```python
from build123d import *

# Parameters (mm, degrees)
SKETCH_R   = 25.426446
SKETCH_R_2 = 1.991345
PAD_DEPTH  = 5


with BuildPart() as part:
    # Sketch → Pad (new body)
    with BuildSketch(Plane.XY):
        Circle(SKETCH_R)
        Circle(SKETCH_R_2, mode=Mode.SUBTRACT)
        with BuildLine():
            Line((-22.250395, 0), (-20.250395, 0))
            ThreePointArc((20.250395, 0), (0, 20.250395), (-20.250395, 0))
            Line((20.250395, 0), (22.250395, 0))
            ThreePointArc((22.250395, 0), (0, 22.250395), (-22.250395, 0))
        make_face(mode=Mode.SUBTRACT)
        with BuildLine():
            ThreePointArc((12.197871, 12.197871), (0, 17.250395), (-12.197871, 12.197871))
            Line((-12.197871, 12.197871), (-10.783657, 10.783657))
            ThreePointArc((10.783657, 10.783657), (0, 15.250395), (-10.783657, 10.783657))
            Line((10.783657, 10.783657), (12.197871, 12.197871))
        make_face(mode=Mode.SUBTRACT)
        with BuildLine():
            Line((10.783657, -10.783657), (12.197871, -12.197871))
            ThreePointArc((-12.197871, -12.197871), (0, -17.250395), (12.197871, -12.197871))
            Line((-12.197871, -12.197871), (-10.783657, -10.783657))
            ThreePointArc((-10.783657, -10.783657), (0, -15.250395), (10.783657, -10.783657))
        make_face(mode=Mode.SUBTRACT)
        with BuildLine():
            ThreePointArc((-4.688023, 11.317889), (-8.662337, 8.662337), (-11.317889, 4.688023))
            Line((-11.317889, 4.688023), (-9.47013, 3.922656))
            ThreePointArc((-3.922656, 9.47013), (-7.248124, 7.248124), (-9.47013, 3.922656))
            Line((-4.688023, 11.317889), (-3.922656, 9.47013))
        make_face(mode=Mode.SUBTRACT)
        with BuildLine():
            ThreePointArc((11.317889, 4.688023), (8.662337, 8.662337), (4.688023, 11.317889))
            Line((4.688023, 11.317889), (3.922656, 9.47013))
            ThreePointArc((9.47013, 3.922656), (7.248124, 7.248124), (3.922656, 9.47013))
            Line((11.317889, 4.688023), (9.47013, 3.922656))
        make_face(mode=Mode.SUBTRACT)
        with BuildLine():
            ThreePointArc((-11.317889, -4.688023), (-8.662337, -8.662337), (-4.688023, -11.317889))
            Line((-4.688023, -11.317889), (-3.922656, -9.47013))
            ThreePointArc((-9.47013, -3.922656), (-7.248124, -7.248124), (-3.922656, -9.47013))
            Line((-11.317889, -4.688023), (-9.47013, -3.922656))
        make_face(mode=Mode.SUBTRACT)
        with BuildLine():
            ThreePointArc((3.922656, -9.47013), (7.248124, -7.248124), (9.47013, -3.922656))
            Line((11.317889, -4.688023), (9.47013, -3.922656))
            ThreePointArc((4.688023, -11.317889), (8.662337, -8.662337), (11.317889, -4.688023))
            Line((4.688023, -11.317889), (3.922656, -9.47013))
        make_face(mode=Mode.SUBTRACT)
        with BuildLine():
            ThreePointArc((0, 7.250395), (-7.250395, 0), (0, -7.250395))
            Line((0, -5.250395), (0, -7.250395))
            ThreePointArc((0, 5.250395), (-5.250395, 0), (0, -5.250395))
            Line((0, 7.250395), (0, 5.250395))
        make_face(mode=Mode.SUBTRACT)
    extrude(amount=PAD_DEPTH)


solid = part.part
```
Model file for the job. Use its own axes, mm. Give positions to 0.01 mm unless a question says otherwise; leave off trailing zeros. Order: outer loops, then holes, each group sorted by start corner. A loop starts at its lowest first (then second) coordinate and runs counter-clockwise, first axis right, second up.
1) Pin check, flat tips, straight feed: pin 1 (3 mm diameter, centred on x = -1, z = 3.5, fed in from +Y); pin 2 (1.6 mm diameter, centred on y = 6.5, z = 3.5, fed in from -X); pin 3 (1 mm diameter, centred on x = -21.5, z = 3, fed in from +Y). Stop position of each tip, or through.
2) Mould opens along X. For faces 1 (the cylindrical face through (7.288, 7.208, 2.465)), 2 (the cylindrical face through (24.25, 7.64, 2.46)) say: +X half, -X half, draft (parallel to the pull), parting line (faces both ways), or undercut.
3) Wall check: probe 1 along X at (y, z) = (-4.5, 1.15); probe 2 along X at (y, z) = (-9, 3); probe 3 along X at (y, z) = (9, 0.65). Give the ranges that are in metal, low to high.
4) Saw through at B-B, the plane z = 2.4. Count the separate pieces of the cut face and the enclosed holes in it, then the cut area to 3 significant figures.
5) Saw through at D-D, the plane x = 14. Write the cut outline in (y, z).
6) Saw through at C-C, the plane y = 6. Write the cut outline in (x, z), then the cut area to 3 significant figures.
7) Saw through at A-A, the plane x = -1. Write the cut outline in (y, z).
Computed:
1. pin 1: stops at y = 25.43
1. pin 2: stops at x = -24.78
1. pin 3: stops at y = 14.34
2. face 1: undercut
2. face 2: parting line
3. probe 1: x = -25.03 to -10.86, -9.21 to -5.68, -2.7 to 9.21, 10.86 to 25.03
3. probe 2: x = -23.78 to -8.31, -4.91 to 4.91, 8.31 to 23.78
3. probe 3: x = -23.78 to -20.35, -18.14 to -8.31, -4.91 to 4.91, 8.31 to 18.14, 20.35 to 23.78
4. separate pieces: 1
4. enclosed holes: 9
4. area: 1,670 mm2
5. outline: (-21.23, 0) - (14.63, 0) - (14.63, 5) - (-21.23, 5) - close; (17.29, 0) - (21.23, 0) - (21.23, 5) - (17.29, 5) - close
6. outline: (-24.71, 0) - (-21.43, 0) - (-21.43, 5) - (-24.71, 5) - close; (-19.34, 0) - (-10.68, 0) - (-10.68, 5) - (-19.34, 5) - close; (-8.31, 0) - (-4.07, 0) - (-4.07, 5) - (-8.31, 5) - close; (0, 0) - (8.31, 0) - (8.31, 5) - (0, 5) - close; (10.68, 0) - (19.34, 0) - (19.34, 5) - (10.68, 5) - close; (21.43, 0) - (24.71, 0) - (24.71, 5) - (21.43, 5) - close
6. area: 182 mm2
7. outline: (-25.41, 0) - (-17.22, 0) - (-17.22, 5) - (-25.41, 5) - close; (-15.22, 0) - (-7.18, 0) - (-7.18, 5) - (-15.22, 5) - close; (-5.15, 0) - (-1.72, 0) - (-1.72, 5) - (-5.15, 5) - close; (1.72, 0) - (5.15, 0) - (5.15, 5) - (1.72, 5) - close; (7.18, 0) - (15.22, 0) - (15.22, 5) - (7.18, 5) - close; (17.22, 0) - (20.23, 0) - (20.23, 5) - (17.22, 5) - close; (22.23, 0) - (25.41, 0) - (25.41, 5) - (22.23, 5) - close
